Geometry check sheet. Reference: the model listing, model coordinates, mm. Face numbers are marked on the shaded views. A direction names the side the tool comes from. Coordinates: 2 decimals unless noted, no trailing zeros. Order: outer loops, then holes, each group sorted by start corner. A loop starts at its lowest first (then second) coordinate and runs counter-clockwise, first axis right, second up. Notation, with made-up numbers: M -31.75,89.25 L 21.25,89.25 A27 ccw 21.25,124.25 Z; hole C 2,-13.5 d7. An arc over 180 degrees is marked long. Use CSV: the item, a comma, the result in double quotes. Start each with the question number.
```python
from build123d import *

# Parameters (mm, degrees)
SKETCH1_W           = 42
SKETCH1_H           = 6
BOSS_EXTRUDE1_DEPTH = 14
BOSS_EXTRUDE2_DEPTH = 14
SKETCH3_R           = 4
CUT_EXTRUDE1_DEPTH  = 14
SKETCH4_R           = 1
CUT_EXTRUDE2_DEPTH  = 14
FILLET1_R           = 1
FILLET2_R           = 1
FILLET3_R           = 1
FILLET4_R           = 1
CHAMFER1_SIZE       = 1
CHAMFER2_SIZE       = 1
CUT_EXTRUDE4_DEPTH  = 14
SKETCH7_R           = 2
CUT_EXTRUDE5_DEPTH  = 24
SKETCH10_W          = 63.901140572
SKETCH10_H          = 43.979020276
CUT_EXTRUDE8_DEPTH  = 2
SKETCH11_W          = 62.872788093
SKETCH11_H          = 44.7095382
CUT_EXTRUDE9_DEPTH  = 2
CHAMFER3_SIZE       = 1
CHAMFER4_SIZE       = 1


with BuildPart() as part:
    # Sketch1 → Boss-Extrude1 (new body)
    with BuildSketch(Plane.XY):
        Rectangle(SKETCH1_W, SKETCH1_H)
    extrude(amount=BOSS_EXTRUDE1_DEPTH)

    # Sketch2 → Boss-Extrude2 (add)
    with BuildSketch(Plane.XY.offset(14)):
        Polygon((0, 28), (-9, 28), (-9, 3), (9, 3), (9, 28), align=None)
    extrude(amount=-BOSS_EXTRUDE2_DEPTH)

    # Sketch3 → Cut-Extrude1 (cut)
    with BuildSketch(Plane.XY.offset(14)):
        with Locations((0, 15)):
            Circle(SKETCH3_R)
    extrude(amount=-CUT_EXTRUDE1_DEPTH, mode=Mode.SUBTRACT)

    # Sketch4 → Cut-Extrude2 (cut)
    with BuildSketch(Plane.XZ.offset(3)):
        with Locations(Location((-16, 7, 0), (0, 0, 270))):
            Circle(SKETCH4_R)
        with Locations(Location((16, 7, 0), (0, 0, 270))):
            Circle(SKETCH4_R)
    extrude(amount=-CUT_EXTRUDE2_DEPTH, mode=Mode.SUBTRACT)

    # Fillet1
    fillet1_edges = [part.edges().sort_by_distance(p)[0] for p in [
        (-9, 3, 7),
    ]]
    fillet(fillet1_edges, radius=FILLET1_R)

    # Fillet2
    fillet2_edges = [part.edges().sort_by_distance(p)[0] for p in [
        (9, 3, 7),
    ]]
    fillet(fillet2_edges, radius=FILLET2_R)

    # Fillet3
    fillet3_edges = [part.edges().sort_by_distance(p)[0] for p in [
        (-9, 28, 7),
    ]]
    fillet(fillet3_edges, radius=FILLET3_R)

    # Fillet4
    fillet4_edges = [part.edges().sort_by_distance(p)[0] for p in [
        (9, 28, 7),
    ]]
    fillet(fillet4_edges, radius=FILLET4_R)

    # Chamfer1
    chamfer1_edges = [part.edges().sort_by_distance(p)[0] for p in [
        (-4, 15, 14),
    ]]
    chamfer(chamfer1_edges, length=CHAMFER1_SIZE)

    # Chamfer2
    chamfer2_edges = [part.edges().sort_by_distance(p)[0] for p in [
        (-4, 15, 0),
    ]]
    chamfer(chamfer2_edges, length=CHAMFER2_SIZE)

    # Sketch6 → Cut-Extrude4 (cut)
    with BuildSketch(Plane.XY.offset(14)):
        with BuildLine():
            Line((0, 28), (-1.5, 28))
            Line((-1.5, 28), (-1.5, 18.708099244))
            ThreePointArc((-1.5, 18.708099244), (0, 19), (1.5, 18.708099244))
            Line((1.5, 18.708099244), (1.5, 28))
            Line((1.5, 28), (0, 28))
        make_face()
    extrude(amount=-CUT_EXTRUDE4_DEPTH, mode=Mode.SUBTRACT)

    # Sketch7 → Cut-Extrude5 (cut)
    with BuildSketch(Plane(origin=(9, 0, 0), x_dir=(0, 0, -1), z_dir=(1, 0, 0))):
        with Locations(Location((-7, 23.5, 0), (0, 0, 90))):
            Circle(SKETCH7_R)
    extrude(amount=-CUT_EXTRUDE5_DEPTH, mode=Mode.SUBTRACT)

    # Sketch10 → Cut-Extrude8 (cut)
    with BuildSketch(Plane.XY.offset(14)):
        with Locations((1.003303608, 14.168104251)):
            Rectangle(SKETCH10_W, SKETCH10_H)
    extrude(amount=-CUT_EXTRUDE8_DEPTH, mode=Mode.SUBTRACT)

    # Sketch11 → Cut-Extrude9 (cut)
    with BuildSketch(Plane(origin=(0, 0, 0), x_dir=(-1, 0, 0), z_dir=(0, 0, -1))):
        with Locations((3.111885471, 13.654031467)):
            Rectangle(SKETCH11_W, SKETCH11_H)
    extrude(amount=-CUT_EXTRUDE9_DEPTH, mode=Mode.SUBTRACT)

    # Chamfer3
    chamfer3_edges = [part.edges().sort_by_distance(p)[0] for p in [
        (0, 11, 12),
    ]]
    chamfer(chamfer3_edges, length=CHAMFER3_SIZE)

    # Chamfer4
    chamfer4_edges = [part.edges().sort_by_distance(p)[0] for p in [
        (0, 11, 2),
    ]]
    chamfer(chamfer4_edges, length=CHAMFER4_SIZE)


solid = part.part
```
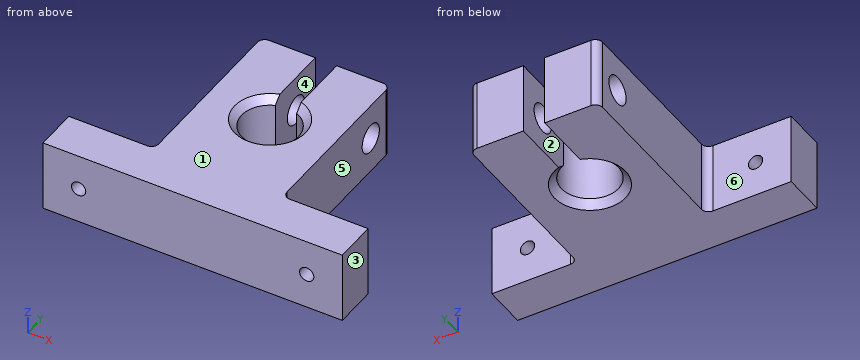
1) Set-up check for the marked faces 4, 5 and 6: record each of +Z, -Z, +X, -X, +Y, -Y from which the full face is reachable in a straight line by a thin tool's end or side.
2) Section check C-C on z = 7. State how many separate pieces and enclosed holes the cut face has, then the cut area to 3 significant figures.
3) Draft check along X on the marked faces 1, 2 and 3. Enter one of: +X half, -X half, draft (parallel to the pull), parting line (faces both ways), or undercut.
4) Section check A-A on y = 15. Record the boundary of the cut face in (x, z), then the cut area to 3 significant figures.
5) Material ranges on line 1 along X through (y, z) = (-1.4, 7); line 2 along X through (y, z) = (15, 6.5); line 3 along X through (y, z) = (20, 10), recorded low to high.
6) Gauge pin test, flat ends, axial feed: P1, Ø1, axis at y = 8, z = 10, coming from the -X side; P2, Ø3, axis at y = 14.5, z = 7, coming from the +X side; P3, Ø2.5, axis at x = -16, z = 7, coming from the +Y side; P4, Ø2.5, axis at y = 23.5, z = 7, coming from the +X side. Record the tip position at first contact, or that the pin passes through.
7) Section check B-B on x = 16. Record the boundary of the cut face in (y, z).
8) Section check D-D on y = 23.5. Record the boundary of the cut face in (x, z), then the cut area to 3 significant figures.
Results are:
1,face 4,"+Z, -Z, +Y"
1,face 5,"+Z, -Z, +X, +Y"
1,face 6,"+Z, -Z, -X, +Y"
2,separate pieces,"5"
2,enclosed holes,"0"
2,area,"540 mm²"
3,face 1,"draft"
3,face 2,"undercut"
3,face 3,"+X half"
4,outline,"M -9,2 L -5,2 L -4,3 L -4,11 L -5,12 L -9,12 Z; M 4,3 L 5,2 L 9,2 L 9,12 L 5,12 L 4,11 Z"
4,area,"98.0 mm²"
5,line 1,"x = -21 to -17, -15 to 15, 17 to 21"
5,line 2,"x = -9 to -4, 4 to 9"
5,line 3,"x = -9 to -1.5, 1.5 to 9"
6,P1,"stops at x = -9"
6,P2,"stops at x = 9"
6,P3,"stops at y = 3"
6,P4,"passes through"
7,outline,"M -3,2 L 3,2 L 3,6 L -3,6 Z; M -3,8 L 3,8 L 3,12 L -3,12 Z"
8,outline,"M -9,2 L -1.5,2 L -1.5,5 L -9,5 Z; M -9,9 L -1.5,9 L -1.5,12 L -9,12 Z; M 1.5,2 L 9,2 L 9,5 L 1.5,5 Z; M 1.5,9 L 9,9 L 9,12 L 1.5,12 Z"
8,area,"90.0 mm²"
